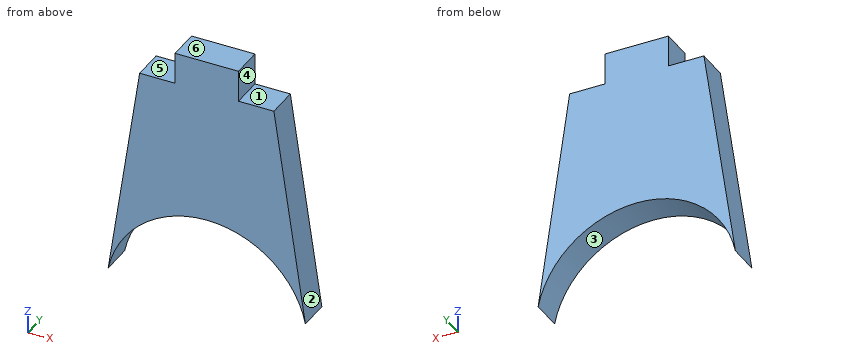
from build123d import *

# Parameters (mm, degrees)
BOSS_EXTRUDE1_DEPTH = 2.5


with BuildPart() as part:
    # Sketch1 → Boss-Extrude1 (new, symmetric)
    with BuildSketch(Plane(origin=(0, 0, 0), x_dir=(-1, 0, 0), z_dir=(0, 1, 0))):
        with BuildLine():
            Line((-5, 37.258597416), (-10.584590832, 37.258597416))
            Line((-10.584590832, 37.258597416), (-15.551383484, 3.189058909))
            ThreePointArc((-15.551383484, 3.189058909), (0, 15.875), (15.551383484, 3.189058909))
            Line((15.551383484, 3.189058909), (10.584590832, 37.258597416))
            Line((10.584590832, 37.258597416), (5, 37.258597416))
            Line((5, 37.258597416), (5, 42.258597416))
            Line((5, 42.258597416), (-5, 42.258597416))
            Line((-5, 42.258597416), (-5, 37.258597416))
        make_face()
    extrude(amount=BOSS_EXTRUDE1_DEPTH, both=True)


solid = part.part
Geometry check sheet. Reference: the model listing, model coordinates, mm. Face numbers are marked on the shaded views. A direction names the side the tool comes from. Give positions to 0.01 mm unless a question says otherwise; leave off trailing zeros. Order: outer loops, then holes, each group sorted by start corner. A loop starts at its lowest first (then second) coordinate and runs counter-clockwise, first axis right, second up. Notation, with made-up numbers: (41, 58) - (100, 58) arc R36 cw to (100, 92) - close; hole circle Ø11 at (12.5, -7). An arc over 180 degrees is marked (long way). Answer as a JSON object with one key per item and string values.
(1) Cross-section at C-C (z = 10). Record the cut outline in (x, y).
Report:
{"outline": "(-14.56, -2.5) - (-12.33, -2.5) - (-12.33, 2.5) - (-14.56, 2.5) - close; (12.33, -2.5) - (14.56, -2.5) - (14.56, 2.5) - (12.33, 2.5) - close"}
(2) Tool access check on the marked faces 4, 5 and 6. Record the directions out of +Z, -Z, +X, -X, +Y, -Y that give a thin tool (end or side, any length) a straight path to the whole face; none if there is none.
Report:
{"face 4": "+Z, +X, +Y, -Y", "face 5": "+Z, -X, +Y, -Y", "face 6": "+Z, +X, -X, +Y, -Y"}
(3) Cross-section at B-B (y = 0.6). Record the cut outline in (x, z) (3 decimals).
Report:
{"outline": "(-15.551, 3.189) arc R15.875 cw to (15.551, 3.189) - (10.585, 37.259) - (5, 37.259) - (5, 42.259) - (-5, 42.259) - (-5, 37.259) - (-10.585, 37.259) - close"}
(4) Depth check by flat-ended pin: pin 1 Ø1.5 at (y, z) = (0.5, 24) entering from -X; pin 2 Ø1 at (x, y) = (-12, -1.5) entering from -Z; pin 3 Ø2.5 at (x, y) = (-9, 0.5) entering from +Z; pin 4 Ø1.5 at (x, z) = (-7.5, 12.5) entering from +Y. Enter the tip coordinate at first touch or a pass-through.
Report:
{"pin 1": "x = -12.63", "pin 2": "z = 9.79", "pin 3": "z = 37.26", "pin 4": "through"}
(5) Draft check along X on the marked faces 1, 2 and 3. Enter one of: released by +X, released by -X, zero draft, split by the parting line, or undercut.
Report:
{"face 1": "zero draft", "face 2": "released by +X", "face 3": "undercut"}
(6) Cross-section at D-D (z = 39.5). Record the cut outline in (x, y).
Report:
{"outline": "(-5, -2.5) - (5, -2.5) - (5, 2.5) - (-5, 2.5) - close"}
(7) Cross-section at A-A (z = 15). Record the cut outline in (x, y).
Report:
{"outline": "(-13.83, -2.5) - (-5.2, -2.5) - (-5.2, 2.5) - (-13.83, 2.5) - close; (5.2, -2.5) - (13.83, -2.5) - (13.83, 2.5) - (5.2, 2.5) - close"}
(8) Material ranges on line 1 (X direction, y = 0.65, z = 39.5); line 2 (Z direction, x = 0.5, y = -0.6); line 3 (X direction, y = 0.95, z = 9.5), recorded low to high.
Report:
{"line 1": "-5 to 5", "line 2": "15.87 to 42.26", "line 3": "-14.63 to -12.72, 12.72 to 14.63"}
